Autodesk Inventor part; units mm, degrees
ref_plane "YZ Plane" through (0, 0, 0) normal (1, 0, 0) x (0, 1, 0)
ref_plane "XZ Plane" through (0, 0, 0) normal (0, 1, 0) x (-1, 0, 0)
ref_plane "XY Plane" through (0, 0, 0) normal (0, 0, 1) x (1, 0, 0)
sketch "Sketch1" plane through (0, 0, 0) normal (0, 0, 1) x (1, 0, 0)
  line L0 (0, 118.387006) -> (0, -122.322035)
  line L1 (-200.109041, 0) -> (200.109041, 0)
  line L2 (-139, 84) -> (139, 84)
  line L3 (139, 84) -> (139, -65)
  line L4 (120, -84) -> (-120, -84)
  line L5 (-139, -65) -> (-139, 84)
  arc A0 (-139, -65) -> (-120, -84) centre (-120, -65) ccw
  arc A1 (120, -84) -> (139, -65) centre (120, -65) ccw
  point P0 (0, 0)
  dimension "d0" = 278
  dimension "d1" = 168
  dimension "d2" = 19
extrude "Extrusion1" add sketch "Sketch1" against normal blind 10
sketch "Sketch2" plane through (0, 0, -10) normal (0, 0, -1) x (-1, 0, 0)
  line L0 (139, -65) -> (139, 84)
  line L1 (139, 84) -> (-139, 84)
  line L2 (-139, 84) -> (-139, -65)
  arc A0 (-139, -65) -> (-120, -84) centre (-120, -65) ccw
  line L3 (-120, -84) -> (120, -84)
  arc A1 (120, -84) -> (139, -65) centre (120, -65) ccw
  line L4 (-139, 84) -> (-139, 105)
  line L5 (-139, 105) -> (-188, 105)
  line L6 (-189, 106) -> (-189, 133.585786)
  line L7 (-188.707107, 134.292893) -> (-154.292893, 168.707107)
  line L8 (-153.585786, 169) -> (-115, 169)
  line L9 (-114, 168) -> (-114, 89)
  line L10 (-14, 89) -> (-14, 168)
  line L11 (-13, 169) -> (27, 169)
  line L12 (37, 159) -> (37, 144)
  line L13 (42, 139) -> (113, 139)
  line L14 (139, 84) -> (139, 104)
  line L15 (189, 104) -> (189, 135)
  line L16 (189, 135) -> (155, 169)
  line L17 (155, 169) -> (132, 169)
  arc A2 (-114, 89) -> (-109, 84) centre (-109, 89) ccw
  arc A3 (-19, 84) -> (-14, 89) centre (-19, 89) ccw
  arc A4 (-188.707107, 134.292893) -> (-189, 133.585786) centre (-188, 133.585786) ccw
  arc A5 (-189, 106) -> (-188, 105) centre (-188, 106) ccw
  arc A6 (-153.585786, 169) -> (-154.292893, 168.707107) centre (-153.585786, 168) ccw
  arc A7 (-114, 168) -> (-115, 169) centre (-115, 168) ccw
  arc A8 (-13, 169) -> (-14, 168) centre (-13, 168) ccw
  arc A9 (113, 139) -> (127, 153) centre (113, 153) ccw
  arc A10 (37, 144) -> (42, 139) centre (42, 144) ccw
  line L18 (127, 164) -> (127, 153)
  line L19 (139, 104) -> (189, 104)
  circle A11 centre (27, 159) radius 6
  arc A12 (37, 159) -> (27, 169) centre (27, 159) ccw
  line L20 (132, 169) -> (127, 164)
  line L21 (-139, 84) -> (-135, 84)
  line L22 (-139, 84) -> (-109, 84)
  line L23 (-139, 84) -> (139, 84)
  line L24 (-19, 84) -> (139, 84)
  point P0 (0, 0)
  point P1 (-189, 105)
  point P2 (-154, 169)
  point P3 (-14, 169)
  point P4 (37, 139)
  point P5 (127, 139)
  point P6 (127, 169)
  point P7 (135, 84)
  dimension "d8" = 21
  dimension "d9" = 50
  dimension "d10" = 85
  dimension "d11" = 75
  dimension "d12" = 135
  dimension "d13" = 40
  dimension "d14" = 100
  dimension "d16" = 90
  dimension "d17" = 50
  dimension "d19" = 34
  dimension "d20" = 135
  dimension "d21" = 5
  dimension "d22" = 1
  dimension "d23" = 14
  dimension "d24" = 5
  dimension "d26" = 90
  dimension "d29" = 12
  dimension "d30" = 226
  dimension "d31" = 5
  dimension "d32" = 5
  dimension "d33" = 55
  dimension "d34" = 20
  dimension "d35" = 16
  dimension "d36" = 75
  dimension "d37" = 112
  dimension "d38" = 26
extrude "Extrusion2" add sketch "Sketch2" against normal blind 10 contours L1 A3 L10 A8 L11 A12 L12 A10 L13 A9 L18 L20 L17 L16 L15 L19 L14 | L1 L4 L5 A5 L6 A4 L7 A6 L8 A7 L9 A2
chamfer "Chamfer2" distance 4 angle 45 6 edges at (139, 20, -10) (133.435, -78.435, -10) (0, -84, -10) (-133.435, -78.435, -10) (-139, 19.5, -10) (-164, 104, -10)
chamfer "Chamfer3" distance 4 angle 45 1 edges at (-164, 104, 0)
sketch "Sketch3" plane through (189, 106, -10) normal (1, 0, 0) x (0, 0, -1)
  line L0 (0, 27.585786) -> (0, 0)
  line L1 (0, 27.585786) -> (-10, 27.585786)
  line L2 (-10, 0) -> (-10, 27.585786)
  line L3 (0, 0) -> (-10, 0)
  line L4 (0, 0) -> (0, -1)
  line L5 (0, 0) -> (-10, 0)
  line L6 (-10, -1) -> (-10, 0)
  line L7 (0, -1) -> (-10, -1)
  line L8 (-10, 3) -> (-6, -1)
  line L9 (-10, 3) -> (-10, -1)
  line L10 (0, -1) -> (-10, -1)
  line L11 (-10, -1) -> (-6, -1)
  line L12 (-5, -1) -> (-5, 5.993177)
  line L13 (0, -1) -> (0, 0)
  line L14 (0, 3) -> (-4, -1)
  line L15 (0, 3) -> (0, -1)
  line L16 (0, -1) -> (-4, -1)
  point P0 (-10, -106)
  point P1 (-10, 3)
  point P2 (0, 3)
  dimension "d47" = 45
  dimension "d48" = 4
extrude "Extrusion3" cut sketch "Sketch3" against normal up to surface (50 mm away) contours L0 L3 L14 | L4 L7 L14 L3 | L8 L3 L2 | L3 L8 L7 L6
ref_plane "Work Plane1" through (139, 109, -10) normal (-0.5773503, 0.5773503, 0.5773503) x (-0.7071068, -0.7071068, 0)
sketch "Sketch4" plane through (139, 109, -10) normal (-0.5773503, 0.5773503, 0.5773503) x (-0.7071068, -0.7071068, 0)
  line L0 (2.828427, 4.898979) -> (-31.819805, 24.903146)
  line L1 (5.656854, 0) -> (2.828427, 4.898979)
  line L2 (-35.355339, 20.412415) -> (0, 0)
  line L3 (2.828427, 4.898979) -> (0, 0)
  line L4 (0, 0) -> (5.656854, 0)
  line L5 (5.656854, 0) -> (2.828427, 4.898979)
  point P0 (175.362482, -4.082483)
extrude "Extrusion4" cut sketch "Sketch4" against normal blind 10
move faces "Move1" translate (0, 1, 0) faces at (-172.333333, 104, -4.666667) (-155.666667, 105.333333, -2.666667) (-154.333333, 106.666667, -8.666667)
properties part number "SlipersLåda 211018003"
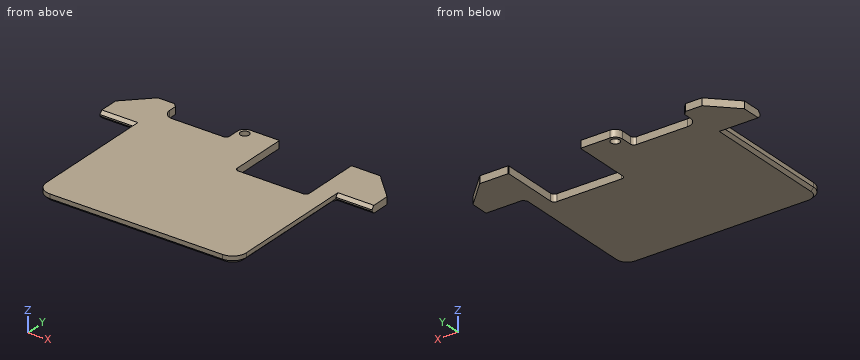
The listing builds one solid part. Answer for the finished solid, in the listing's coordinates (mm). Coordinates: 2 decimals unless noted, no trailing zeros. Order: outer loops, then holes, each group sorted by start corner. A loop starts at its lowest first (then second) coordinate and runs counter-clockwise, first axis right, second up.
Q1. A cutting plane is placed at B-B, the plane y = -15.5. Write down the section's boundary in (x, z), and give its area (3 significant figures).
Q2. Given P1, Ø2, axis at x = 158, z = -4.5, coming from the -Y side; P2, Ø5, axis at y = 158, z = -7, coming from the +X side; P3, Ø12, axis at x = -35, y = 15.5, coming from the +Z side; P4, Ø5, axis at x = 28, z = -2, coming from the +Y side, each flat-ended and moving along its own axis, determine where each tip first touches the part or whether it passes through.
Q3. A cutting plane is placed at A-A, the plane y = 94.5. Write down the section's boundary in (x, z), and give its area (3 significant figures).
Q4. Consider line 1 (Y direction, x = -27, z = -4.5); line 2 (X direction, y = 90, z = -3.5); line 3 (Y direction, x = -29, z = -3). Determine where each line is inside the solid, lowest interval first.
Answers follow:
1. outline: (-139, -6) - (-135, -10) - (135, -10) - (139, -6) - (139, 0) - (-139, 0) - close
1. area: 2,760 mm2
2. P1: stops at y = 105
2. P2: stops at x = 167.5
2. P3: stops at z = 0
2. P4: stops at y = 84
3. outline: (-139, -6) - (-135, -10) - (14, -10) - (14, 0) - (-139, 0) - close; (114, -10) - (135, -10) - (139, -6) - (139, 0) - (114, 0) - close
3. area: 1,760 mm2
4. line 1: y = -84 to 153, 165 to 169
4. line 2: x = -139 to 14, 114 to 139
4. line 3: y = -84 to 153.34, 164.66 to 168.8
